Can you work these out from the model? Positions are in its coordinate system, mm. A direction names the side the tool comes from. Coordinates: 2 decimals unless noted, no trailing zeros. Order: outer loops, then holes, each group sorted by start corner. A loop starts at its lowest first (then second) coordinate and runs counter-clockwise, first axis right, second up. Notation, with made-up numbers: (-24.5, 12) - (-2.5, 12) arc R20 cw to (-2.5, 44) - close; hole circle Ø1 at (-33.75, -16). An arc over 180 degrees is marked (long way). Return JSON: item names as keys, results as strings. Group by question number.
1) For pin 1 Ø4 at (x, z) = (92.5, 243) entering from +Y, with a flat end and sliding along its axis, tell me the tip position at first contact or that it passes through.
2) Imagine slicing it at B-B (x = 211.5). Write out the boundary of the cut face in (y, z).
3) If I drill on line 1 along X through (y, z) = (172, -114.5); line 2 along Z through (x, y) = (-862.5, 421); line 3 along Y through (x, z) = (-20.5, -171), over which ranges is the centre line in solid material (lowest first)?
4) Imagine slicing it at A-A (y = 159.5). Write out the boundary of the cut face in (x, z), and give its area (3 significant figures).
5) If we mould it in two halves opening along Z, with no side actions, what happens to faces 4 (the face through (903, 700, 672)), 5 (the face through (-897.954, 666.134, 672.437)), 6 (the face through (903, 345, 721.338))? For each: pulls with the +Z half, pulls with the -Z half, needs draft (parallel to the pull), parting line crosses it, or undercut.
6) Imagine slicing it at C-C (z = -6.5). Write out the boundary of the cut face in (x, y), and give its area (3 significant figures).
7) Which directions (+Z, -Z, +X, -X, +Y, -Y) give clear straight access to the entire face, cutting with the end or side of a thin tool? Please do faces 1 (the face through (-947.254, 345, -129)), 2 (the face through (-897, 345, -78.662)), 3 (the face through (952.746, 345, -129)).
```python
from build123d import *

# Parameters (mm, degrees)
F0_W      = 2000
F0_H      = 1000
F1_DEPTH  = 25
F2_W      = 100
F2_H      = 100
F3_DEPTH  = 700
F4_W      = 100
F4_H      = 100
F5_DEPTH  = 700
F6_W      = 100
F6_H      = 100
F7_DEPTH  = 700
F8_W      = 100
F8_H      = 100
F9_DEPTH  = 700
F10_R     = 25
F11_DEPTH = 1950.001
F12_R     = 25
F13_DEPTH = 1950.001
F14_R     = 25
F15_DEPTH = 1950.001


with BuildPart() as f1:
    # F0 (on Front) → F1 (new body)
    with BuildSketch(Plane.XZ):
        with Locations((2.746239, 271.337836)):
            Rectangle(F0_W, F0_H)
    extrude(amount=F1_DEPTH)

    # F2 (on face) → F3 (join)
    with BuildSketch(Plane(origin=(0, 0, 0), x_dir=(-1, 0, 0), z_dir=(0, 1, 0))):
        with Locations((-902.746239, 671.337836)):
            Rectangle(F2_W, F2_H)
    extrude(amount=F3_DEPTH)

    # F4 (on face) → F5 (join)
    with BuildSketch(Plane(origin=(0, 0, 0), x_dir=(-1, 0, 0), z_dir=(0, 1, 0))):
        with Locations((897.253761, 671.337836)):
            Rectangle(F4_W, F4_H)
    extrude(amount=F5_DEPTH)

    # F6 (on face) → F7 (join)
    with BuildSketch(Plane(origin=(0, 0, 0), x_dir=(-1, 0, 0), z_dir=(0, 1, 0))):
        with Locations((-902.746239, -128.662164)):
            Rectangle(F6_W, F6_H)
    extrude(amount=F7_DEPTH)

    # F8 (on face) → F9 (join)
    with BuildSketch(Plane(origin=(0, 0, 0), x_dir=(-1, 0, 0), z_dir=(0, 1, 0))):
        with Locations((897.253761, -128.662164)):
            Rectangle(F8_W, F8_H)
    extrude(amount=F9_DEPTH)

    # F10 (on face) → F11 (cut, through all)
    with BuildSketch(Plane(origin=(-947.253761, 0, 0), x_dir=(0, -1, 0), z_dir=(-1, 0, 0))):
        with Locations((-641.158521, 671.337836)):
            Circle(F10_R)
    extrude(amount=-F11_DEPTH, mode=Mode.SUBTRACT)

    # F12 (on face) → F13 (cut, through all)
    with BuildSketch(Plane.YZ.offset(952.746239)):
        with Locations((646.280468, -133.296296)):
            Circle(F12_R)
    extrude(amount=-F13_DEPTH, mode=Mode.SUBTRACT)

    # F14 (on face) → F15 (cut, through all)
    with BuildSketch(Plane.YZ.offset(952.746239)):
        with Locations((458.47559, 672.557294)):
            Circle(F14_R)
    extrude(amount=-F15_DEPTH, mode=Mode.SUBTRACT)


solid = f1.part
```
Calculated:
{
 "1": {"pin 1": "y = 0"},
 "2": {"outline": "(-25, -228.66) - (0, -228.66) - (0, 771.34) - (-25, 771.34) - close"},
 "3": {"line 1": "-947.25 to -847.25, 852.75 to 952.75", "line 2": "-178.66 to -78.66, 621.34 to 721.34", "line 3": "-25 to 0"},
 "4": {"outline": "(-947.25, -178.66) - (-847.25, -178.66) - (-847.25, -78.66) - (-947.25, -78.66) - close; (-947.25, 621.34) - (-847.25, 621.34) - (-847.25, 721.34) - (-947.25, 721.34) - close; (852.75, -178.66) - (952.75, -178.66) - (952.75, -78.66) - (852.75, -78.66) - close; (852.75, 621.34) - (952.75, 621.34) - (952.75, 721.34) - (852.75, 721.34) - close", "area": "40,000 mm2"},
 "5": {"face 4": "needs draft", "face 5": "undercut", "face 6": "pulls with the +Z half"},
 "6": {"outline": "(-997.25, -25) - (1002.75, -25) - (1002.75, 0) - (-997.25, 0) - close", "area": "50,000 mm2"},
 "7": {"face 1": "+Z, -Z, -X, +Y", "face 2": "+X, -X, +Y", "face 3": "+Z, -Z, +X, +Y"}
}
